Autodesk Inventor part; units mm, degrees
ref_plane "YZ Plane" through (0, 0, 0) normal (1, 0, 0) x (0, 1, 0)
ref_plane "XZ Plane" through (0, 0, 0) normal (0, 1, 0) x (-1, 0, 0)
ref_plane "XY Plane" through (0, 0, 0) normal (0, 0, 1) x (1, 0, 0)
sketch "スケッチ1" plane through (0, 0, 0) normal (0, 0, 1) x (1, 0, 0)
  line L0 (-25.5, 29) -> (25.5, 29)
  line L1 (25.5, 29) -> (25.5, -29)
  line L2 (25.5, -29) -> (-25.5, -29)
  line L3 (-25.5, -29) -> (-25.5, 29)
  point P0 (0, 0)
  point P1 (-25.5, 0)
  point P2 (0, -29)
  dimension "d0" = 51
  dimension "d1" = 58
extrude "押し出し1" add sketch "スケッチ1" along normal blind 14.5
fillet "フィレット1" radius 6 4 edges at (0, 29, 14.5) (0, 29, 0) (0, -29, 14.5) (0, -29, 0)
properties part number "AA-Cellx4"
For this review, take the finished solid that the model builds, in its own axes (mm). Round coordinates to 2 decimals unless told otherwise and drop trailing zeros. Write each loop counter-clockwise with the first axis right and the second up, starting at its lowest first coordinate (ties: lowest second). Pieces come first, ordered by that corner, then holes. Notation, with made-up numbers: (81, -1) - (120, -1) arc R10 ccw to (120, 16) - close; hole circle Ø11 at (57.25, 68). An arc over 180 degrees is marked (long way). Write item = value, one per line. Start each with the question number.
1. For pin 1 Ø4 at (x, z) = (7.5, 3) entering from +Y, flat-tipped, find the tip position at first contact; note if it passes through.
2. Wall thickness on L1, parallel to Y at x = 13, z = 11.25; L2, parallel to Y at x = -8.5, z = 4.75; L3, parallel to Z at x = -16, y = 25: over which ranges is each line inside the solid? List them lowest first.
3. Consider section B-B on z = 13. State the section outline as (x, y) points.
4. Consider section A-A on x = 22.5. State the section outline as (y, z) points, plus the area to 3 significant figures.
5. Consider section C-C on y = -25. State the section outline as (x, z) points.
Evaluation:
q1.pin_1 = 28.92
q2.L1 = -28.33 to 28.33
q2.L2 = -28.87 to 28.87
q2.L3 = 0.34 to 14.16
q3.outline = (-25.5, -26.97) - (25.5, -26.97) - (25.5, 26.97) - (-25.5, 26.97) - close
q4.outline = (-29, 6) arc R6 ccw to (-23, 0) - (23, 0) arc R6 ccw to (29, 6) - (29, 8.5) arc R6 ccw to (23, 14.5) - (-23, 14.5) arc R6 ccw to (-29, 8.5) - close
q4.area = 810 mm2
q5.outline = (-25.5, 0.34) - (25.5, 0.34) - (25.5, 14.16) - (-25.5, 14.16) - close
